Design review of the part built by this model. Coordinates are the model's own, in mm. A direction names the side the tool comes from. Coordinates: 2 decimals unless noted, no trailing zeros. Write each loop counter-clockwise with the first axis right and the second up, starting at its lowest first coordinate (ties: lowest second). Pieces come first, ordered by that corner, then holes. Notation, with made-up numbers: (24, 29) - (61, 29) arc R11 cw to (61, 39) - close; hole circle Ø4 at (66.5, 3). An arc over 180 degrees is marked (long way). Use a Markdown table: item, result.
from build123d import *

# Parameters (mm, degrees)
SKETCH1_W           = 142.3995226
SKETCH1_H           = 44
SKETCH1_R           = 2
BOSS_EXTRUDE1_DEPTH = 2.5
FILLET1_R           = 4


with BuildPart() as part:
    # Sketch1 → Boss-Extrude1 (new body)
    with BuildSketch(Plane(origin=(0, 0, 0), x_dir=(1, 0, 0), z_dir=(0, 1, 0))):
        Rectangle(SKETCH1_W, SKETCH1_H)
        with Locations(Location((-65.1997613, 16, 0), (0, 0, 270))):
            Circle(SKETCH1_R, mode=Mode.SUBTRACT)
        with Locations(Location((65.1997613, 16, 0), (0, 0, 270))):
            Circle(SKETCH1_R, mode=Mode.SUBTRACT)
        with Locations(Location((65.1997613, -16, 0), (0, 0, 270))):
            Circle(SKETCH1_R, mode=Mode.SUBTRACT)
        with Locations(Location((-65.1997613, -16, 0), (0, 0, 270))):
            Circle(SKETCH1_R, mode=Mode.SUBTRACT)
        Polygon((-61.1997613, 16), (-61.1997613, -16), (-13.733525191, 16), align=None, mode=Mode.SUBTRACT)
        Polygon((-3, 16), (-50.466236109, -16), (-3, -16), align=None, mode=Mode.SUBTRACT)
        Polygon((3, 16), (3, -16), (50.466236109, -16), align=None, mode=Mode.SUBTRACT)
        Polygon((61.1997613, -16), (13.733525191, 16), (61.1997613, 16), align=None, mode=Mode.SUBTRACT)
    extrude(amount=BOSS_EXTRUDE1_DEPTH)

    # Fillet1
    fillet1_edges = [part.edges().sort_by_distance(p)[0] for p in [
        (-13.733525191, 1.25, -16),
        (-61.1997613, 1.25, -16),
        (-61.1997613, 1.25, 16),
        (-3, 1.25, 16),
        (-3, 1.25, -16),
        (-50.466236109, 1.25, 16),
        (50.466236109, 1.25, 16),
        (3, 1.25, -16),
        (3, 1.25, 16),
        (61.1997613, 1.25, 16),
        (61.1997613, 1.25, -16),
        (13.733525191, 1.25, -16),
        (-71.1997613, 1.25, -22),
        (71.1997613, 1.25, -22),
        (71.1997613, 1.25, 22),
        (-71.1997613, 1.25, 22),
    ]]
    fillet(fillet1_edges, radius=FILLET1_R)


solid = part.part
(1) Take a section at D-D on y = 1.85. State how many separate pieces and enclosed holes the cut face has, and give its area (3 significant figures).
Determined:
| item | result |
|---|---|
| separate pieces | 1 |
| enclosed holes | 8 |
| area | 3,360 mm2 |
(2) Take a section at A-A on x = -35. Write out the cut boundary in (y, z).
Determined:
| item | result |
|---|---|
| outline | (0, -22) - (2.5, -22) - (2.5, -16) - (0, -16) - close; (0, -1.66) - (2.5, -1.66) - (2.5, 5.57) - (0, 5.57) - close; (0, 16) - (2.5, 16) - (2.5, 22) - (0, 22) - close |
(3) Take a section at C-C on x = -17. Write out the cut boundary in (y, z), and give its area (3 significant figures).
Determined:
| item | result |
|---|---|
| outline | (0, -22) - (2.5, -22) - (2.5, -6.56) - (0, -6.56) - close; (0, 16) - (2.5, 16) - (2.5, 22) - (0, 22) - close |
| area | 53.6 mm2 |
(4) For L1, parallel to X at y = 1.6, z = 13; L2, parallel to Z at x = 30, y = 1.55; L3, parallel to Z at x = 64, y = 1.7, list the stretches that pass through material, from the lowest coordinate up. Write a range as from..to.
Determined:
| item | result |
|---|---|
| L1 | -71.2..-41.25, -3.13..3.13, 41.25..71.2 |
| L2 | -22..-16, -5.03..2.2, 16..22 |
| L3 | -22..-17.6, -14.4..14.4, 17.6..22 |
(5) Draft analysis for pull direction X (two halves, no side actions). For faces 3 (the flat face through (-71.2, 1, 0)), 4 (the flat face through (-1, 1, 22)), 5 (the flat face through (22, 1, 16)), 6 (the flat face through (39.99, 1.23, 1.7)), state which applies: +X half, -X half, draft (parallel to the pull), parting line (faces both ways), or undercut.
Determined:
| item | result |
|---|---|
| face 3 | -X half |
| face 4 | draft |
| face 5 | undercut |
| face 6 | undercut |
(6) Machinability: for faces 1 (the flat face through (-1, 1, -22)), 2 (the cylindrical face through (-41.223, 1.268, 13.101)), which of the approach directions +Z, -Z, +X, -X, +Y, -Y give a long, thin tool a straight path to every point of the face, cutting with its end or side? Answer none if there is none.
Determined:
| item | result |
|---|---|
| face 1 | -Z, +X, -X, +Y, -Y |
| face 2 | +Y, -Y |
(7) Take a section at B-B on z = 1. Write out the cut boundary in (x, y), and give its area (3 significant figures).
Determined:
| item | result |
|---|---|
| outline | (-71.2, 0) - (-61.2, 0) - (-61.2, 2.5) - (-71.2, 2.5) - close; (-38.95, 0) - (-28.22, 0) - (-28.22, 2.5) - (-38.95, 2.5) - close; (-3, 0) - (3, 0) - (3, 2.5) - (-3, 2.5) - close; (28.22, 0) - (38.95, 0) - (38.95, 2.5) - (28.22, 2.5) - close; (61.2, 0) - (71.2, 0) - (71.2, 2.5) - (61.2, 2.5) - close |
| area | 119 mm2 |
